For this review, use the dimensioned drawing (mm, ordinates from the lowest corner) and the shaded views. A direction names the side the tool comes from. Round coordinates to 2 decimals unless told otherwise and drop trailing zeros. Order: outer loops, then holes, each group sorted by start corner. A loop starts at its lowest first (then second) coordinate and runs counter-clockwise, first axis right, second up. Notation, with made-up numbers: M 19,-21.75 L 34,-21.75 A18 ccw 34,-14.75 Z; hole C -17,20.25 d3. An arc over 180 degrees is marked long. Use a Markdown table: item, result. Add a question column.
1. Consider section A-A on y = 14.75. State the section outline as (x, z) points (3 decimals), then the cut area to 3 significant figures.
2. Consider section B-B on z = 8.25. State the section outline as (x, y) points, then the cut area to 3 significant figures.
3. Consider section D-D on y = 23.75. State the section outline as (x, z) points, then the cut area to 3 significant figures.
4. For the marked faces 4, 5 and 6, list the 3-axis set-ups (+Z, -Z, +X, -X, +Y, -Y) from which the entire face can be reached by the end or side of a thin tool; tool diameter is ignored.
5. Consider section C-C on x = 19. State the section outline as (y, z) points.
6. Insertion check: P1, Ø12, axis at x = 15.875, y = 14.75, coming from the -Z side; P2, Ø0.8, axis at y = 14.5, z = 0.5, coming from the -X side; P3, Ø0.8, axis at y = 27.5, z = 9.5, coming from the +X side; P4, Ø4, axis at x = 50, y = 20, coming from the +Z side. Each pin has a flat end and moves straight along its axis. Give the tip position at first contact, or say it passes through.
7. To check wall thickness, follow probe 1 along X at (y, z) = (9, 6); probe 2 along Y at (x, z) = (13, 3.75); probe 3 along Z at (x, y) = (2.5, 27). State the ranges of each line that lie inside material, in increasing order.
8. The part is to be moulded in two halves that separate along Y. For the marked faces 1, 2 and 3, say which applies: +Y half, -Y half, draft (parallel to the pull), parting line (faces both ways), or undercut.
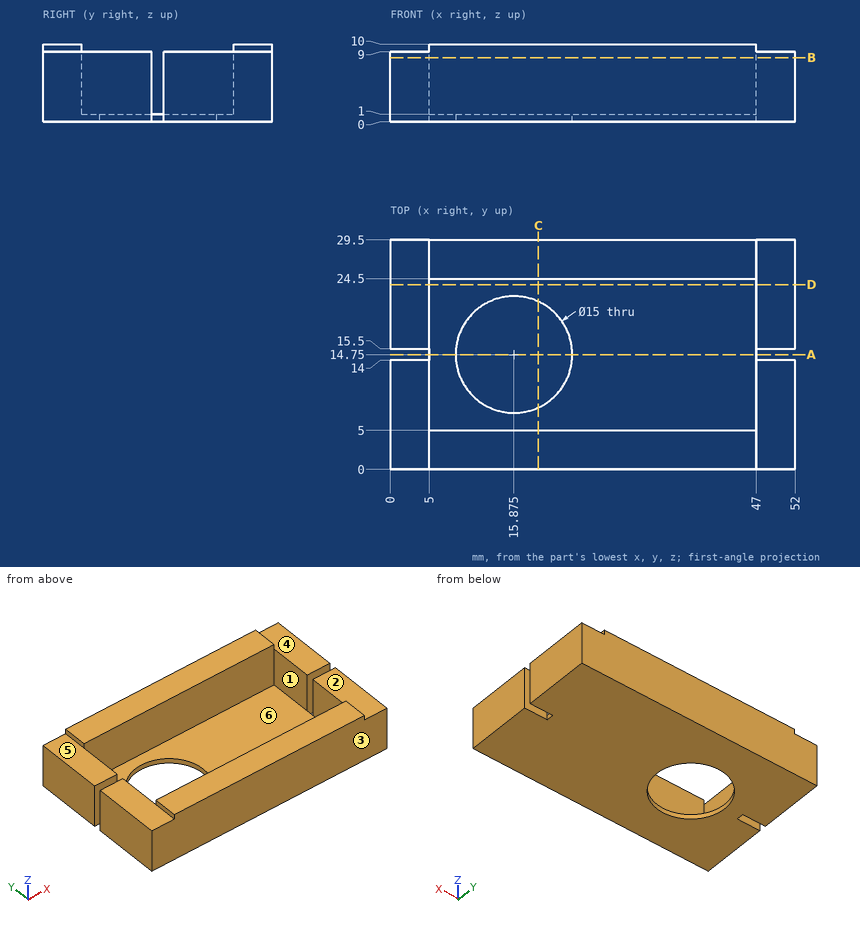
Answer block:
| question | item | result |
|---|---|---|
| 1 | outline | M 5,0 L 8.375,0 L 8.375,1 L 5,1 Z; M 23.375,0 L 47,0 L 47,1 L 23.375,1 Z |
| 1 | area | 27.0 mm^2 |
| 2 | outline | M 0,0 L 52,0 L 52,14 L 47,14 L 47,5 L 5,5 L 5,14 L 0,14 Z; M 0,15.5 L 5,15.5 L 5,24.5 L 47,24.5 L 47,15.5 L 52,15.5 L 52,29.5 L 0,29.5 Z |
| 2 | area | 700 mm^2 |
| 3 | outline | M 0,0 L 52,0 L 52,9 L 47,9 L 47,1 L 5,1 L 5,9 L 0,9 Z |
| 3 | area | 132 mm^2 |
| 4 | face 4 | +Z, +X, +Y, -Y |
| 4 | face 5 | +Z, -X, +Y, -Y |
| 4 | face 6 | +Z |
| 5 | outline | M 0,0 L 7.93,0 L 7.93,1 L 5,1 L 5,10 L 0,10 Z; M 21.57,0 L 29.5,0 L 29.5,10 L 24.5,10 L 24.5,1 L 21.57,1 Z |
| 6 | P1 | through |
| 6 | P2 | x = 5 |
| 6 | P3 | x = 47 |
| 6 | P4 | z = 9 |
| 7 | probe 1 | 0 to 5, 47 to 52 |
| 7 | probe 2 | 0 to 5, 24.5 to 29.5 |
| 7 | probe 3 | 0 to 9 |
| 8 | face 1 | undercut |
| 8 | face 2 | draft |
| 8 | face 3 | -Y half |
